The drawing under review shows one solid part. Ordinate dimensions are in mm from its lowest x, y, z. A direction names the side the tool comes from. Coordinates: 2 decimals unless noted, no trailing zeros. Write each loop counter-clockwise with the first axis right and the second up, starting at its lowest first coordinate (ties: lowest second). Pieces come first, ordered by that corner, then holes.
1) Add section C-C, the plane x = 26. State the section outline as (y, z) points.
2) Add section A-A, the plane y = 15.3. State the section outline as (x, z) points (3 decimals).
3) Mouldability with a two-part tool opening along X and no side actions: class the marked faces 5, 6 and 7 as released by +X, released by -X, zero draft, split by the parting line, or undercut.
4) For line 1 (X direction, y = 12.5, z = 10.5); line 2 (X direction, y = 16.5, z = 8.5) (3 decimals); line 3 (Z direction, x = 61, y = 27), list the stretches that pass through material, from the lowest coordinate up.
5) Add section B-B, the plane z = 17.5. State the section outline as (x, y) points.
6) For P1, Ø3, axis at x = 32, z = 7, coming from the -Y side; P2, Ø8, axis at x = 100, z = 29.5, coming from the +Y side; P3, Ø6, axis at y = 10.5, z = 15.5, coming from the -X side; P4, Ø5, axis at x = 81.5, y = 17, coming from the +Z side, all flat-tipped, find the tip position at first contact; note any pin that passes through.
7) Add section D-D, the plane x = 65.5. State the section outline as (y, z) points.
8) Machinability: for the marked faces 1, 2, 3 and 4, which of the approach directions +Z, -Z, +X, -X, +Y, -Y give a long, thin tool a straight path to every point of the face, cutting with its end or side? Answer none if there is none.
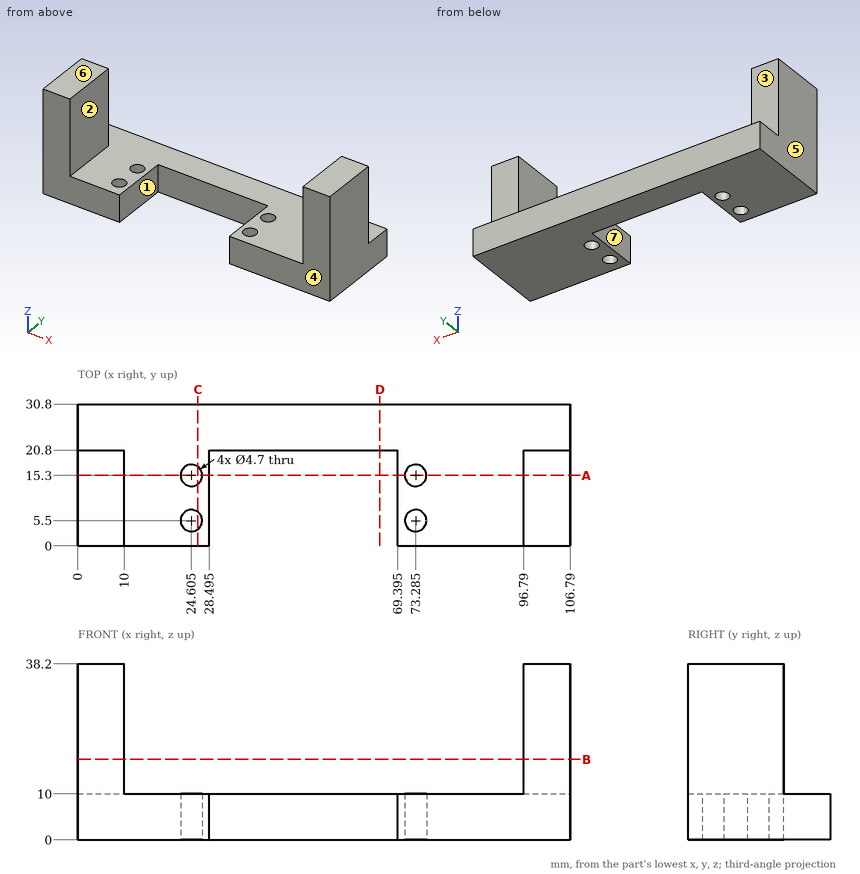
Geometry results:
1. outline: (0, 0) - (3.61, 0) - (3.61, 10) - (0, 10) - close; (7.39, 0) - (13.41, 0) - (13.41, 10) - (7.39, 10) - close; (17.19, 0) - (30.8, 0) - (30.8, 10) - (17.19, 10) - close
2. outline: (0, 0) - (22.255, 0) - (22.255, 10) - (10, 10) - (10, 38.2) - (0, 38.2) - close; (26.955, 0) - (28.495, 0) - (28.495, 10) - (26.955, 10) - close; (69.395, 0) - (70.935, 0) - (70.935, 10) - (69.395, 10) - close; (75.635, 0) - (106.79, 0) - (106.79, 38.2) - (96.79, 38.2) - (96.79, 10) - (75.635, 10) - close
3. face 5: released by -X
3. face 6: zero draft
3. face 7: undercut
4. line 1: x = 0 to 10, 96.79 to 106.79
4. line 2: x = 0 to 22.584, 26.626 to 28.495, 69.395 to 71.264, 75.306 to 106.79
4. line 3: z = 0 to 10
5. outline: (0, 0) - (10, 0) - (10, 20.8) - (0, 20.8) - close; (96.79, 0) - (106.79, 0) - (106.79, 20.8) - (96.79, 20.8) - close
6. P1: stops at y = 20.8
6. P2: stops at y = 20.8
6. P3: stops at x = 0
6. P4: stops at z = 10
7. outline: (20.8, 0) - (30.8, 0) - (30.8, 10) - (20.8, 10) - close
8. face 1: +Z, -Z, -Y
8. face 2: +Z, +Y, -Y
8. face 3: +Z, +X, -X, +Y
8. face 4: +Z, -Z, +X, -X, -Y
